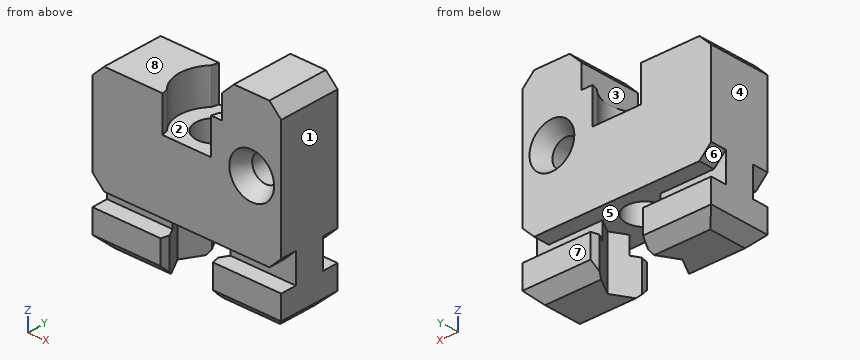
from build123d import *
from OCP.BRepFilletAPI import BRepFilletAPI_MakeChamfer

# Parameters (mm, degrees)
SKETCH1_R           = 1.15
BOSS_EXTRUDE1_DEPTH = 2.6
BOSS_EXTRUDE2_DEPTH = 16
SKETCH3_R           = 1.6
CUT_EXTRUDE1_DEPTH  = 24.13028318
SKETCH4_R           = 3
CUT_EXTRUDE2_DEPTH  = 3
CUT_EXTRUDE3_REACH  = 25.13
CHAMFER1_SIZE       = 0.549227511
CHAMFER1_SIZE_2     = 0.549038106
CHAMFER1_SIZE_3     = 0.75
CHAMFER2_SIZE       = 1
CHAMFER3_SIZE       = 0.75
CHAMFER3_SIZE2      = 1.299038106


with BuildPart() as part:
    # Sketch1 → Boss-Extrude1 (new, symmetric)
    with BuildSketch(Plane(origin=(0, 0, 0), x_dir=(1, 0, 0), z_dir=(0, 1, 0))):
        Polygon((0, 0), (16, 0), (16, -12), (11, -12), (11, -9), (0, -9), align=None)
        with Locations(Location((13.5, -6, 0), (0, 0, 270))):
            Circle(SKETCH1_R, mode=Mode.SUBTRACT)
    extrude(amount=BOSS_EXTRUDE1_DEPTH, both=True)

    # Sketch2 → Boss-Extrude2 (add)
    with BuildSketch(Plane.ZY):
        Polygon((-1.5, -1.25), (-1.5, -2.6), (-4.5, -2.6), (-4.5, 2.6), (-1.5, 2.6), (-1.5, 1.25), (0, 1.25), (0, -1.25), align=None)
    extrude(amount=-BOSS_EXTRUDE2_DEPTH)

    # Sketch3 → Cut-Extrude1 (cut, through all)
    with BuildSketch(Plane(origin=(0, 0, -4.5), x_dir=(-1, 0, 0), z_dir=(0, 0, -1))):
        with Locations((-8, 0)):
            Circle(SKETCH3_R)
    extrude(amount=-CUT_EXTRUDE1_DEPTH, mode=Mode.SUBTRACT)

    # Sketch4 → Cut-Extrude2 (cut)
    with BuildSketch(Plane.XY.offset(9)):
        with Locations((8, 0)):
            Circle(SKETCH4_R)
    extrude(amount=-CUT_EXTRUDE2_DEPTH, mode=Mode.SUBTRACT)

    # Cut-Extrude3: up to this face of the body (flat: up to its plane)
    cut_extrude3_end = Plane(part.part.faces().sort_by_distance((8, 1.937058452, 0))[0])
    # Sketch5 → Cut-Extrude3 (cut, up to the picked face)
    with BuildSketch(Plane(origin=(0, 0, -4.5), x_dir=(-1, 0, 0), z_dir=(0, 0, -1)), mode=Mode.PRIVATE) as cut_extrude3_sk1:
        Polygon((-4.824573519, 0), (-6.41228676, 2.75), (-9.58771324, 2.75), (-11.175426481, 0), (-9.58771324, -2.75), (-6.41228676, -2.75), align=None)
    cut_extrude3_tool1 = split(extrude(cut_extrude3_sk1.sketch, amount=-CUT_EXTRUDE3_REACH, mode=Mode.PRIVATE), bisect_by=cut_extrude3_end, keep=Keep.BOTH, mode=Mode.PRIVATE)
    add(cut_extrude3_tool1.solids().sort_by(Axis((8, 0, -4.5), (0, 0, 1)))[0], mode=Mode.SUBTRACT)

    # Chamfer1
    # the kernel refuses this chamfer: 0.75, 0.549227511, 0.549038106 mm, written as the material it takes off along each edge
    with BuildSketch(Plane(origin=(9.496662955, 2.6, 6), x_dir=(0.7827857508590854, -0.6222913049786071, 0), z_dir=(0, 0, 1)), Plane(origin=(6.503337045, -2.6, 6), x_dir=(-0.7827857508590857, 0.6222913049786067, 0), z_dir=(0, 0, 1))) as chamfer1_piece_1:
        with BuildLine():
            Line((0.892781916, 0), (CHAMFER1_SIZE * 0.782785751548, CHAMFER1_SIZE * 0.622291305526))
            Line((CHAMFER1_SIZE * 0.782785751548, CHAMFER1_SIZE * 0.622291305526), (0, 0))
            ThreePointArc((0, 0), (0.458630217, 0.033371738), (0.892781916, 0))
        make_face()
    extrude(amount=5.292721472, mode=Mode.SUBTRACT)
    with BuildSketch(Plane(origin=(9.496662955, -2.6, 6), x_dir=(0.7827857508590856, 0.6222913049786071, 0), z_dir=(0, 0, 1)), Plane(origin=(6.503337045, 2.6, 6), x_dir=(-0.7827857508590856, -0.622291304978607, 0), z_dir=(0, 0, 1))) as chamfer1_piece_2:
        with BuildLine():
            Line((0.892781916, 0), (CHAMFER1_SIZE * 0.782785751548, -CHAMFER1_SIZE * 0.622291305526))
            Line((CHAMFER1_SIZE * 0.782785751548, -CHAMFER1_SIZE * 0.622291305526), (0, 0))
            ThreePointArc((0, 0), (0.458630217, -0.033371738), (0.892781916, 0))
        make_face()
    extrude(amount=5.292721472, mode=Mode.SUBTRACT)
    with BuildSketch(Plane(origin=(6.325684219, -2.6, -6.428762241), x_dir=(-1, 0, 0), z_dir=(0, 0, 1)), Plane(origin=(9.674315781, -2.6, -1.5), x_dir=(1, 0, 0), z_dir=(0, 0, -1)), Plane(origin=(9.674315781, 2.6, -6.428762241), x_dir=(1, 0, 0), z_dir=(0, 0, 1)), Plane(origin=(6.325684219, 2.6, -1.5), x_dir=(-1, 0, 0), z_dir=(0, 0, -1))) as chamfer1_piece_3:
        Polygon((CHAMFER1_SIZE_2, 0), (CHAMFER1_SIZE_3 * 0.5, -CHAMFER1_SIZE_3 * 0.866025403784), (0, 0), align=None)
    extrude(amount=4.928762241, mode=Mode.SUBTRACT)

    # Chamfer2
    chamfer2_edges = [part.edges().sort_by_distance(p)[0] for p in [
        (16, 0, 12),
        (11, 0, 12),
        (0, 0, 9),
        (16, -1.925, 0),
        (16, 1.925, 0),
        (0, -1.925, 0),
        (0, 1.925, 0),
        (2.888323057, -2.6, -4.5),
        (0, 0, -4.5),
        (16, 0, -4.5),
        (2.888323057, 2.6, -4.5),
        (13.111676943, -2.6, -4.5),
        (13.111676943, 2.6, -4.5),
    ]]
    chamfer(chamfer2_edges, length=CHAMFER2_SIZE)

    # Chamfer3: one chamfer whose edges measure the first distance from different faces: ONE call of the kernel's chamfer builder (chamfer() names one face for all edges)
    chamfer3_edges_1 = [part.edges().sort_by_distance(p)[0] for p in [
        (13.5, -2.6, 4.85),
    ]]
    chamfer3_side_1 = [part.faces().sort_by_distance(p)[0] for p in [
        (8.413951701, -2.6, 4.798840105),
    ]]
    chamfer3_edges_2 = [part.edges().sort_by_distance(p)[0] for p in [
        (13.5, 2.6, 4.85),
    ]]
    chamfer3_side_2 = [part.faces().sort_by_distance(p)[0] for p in [
        (8.413951701, 2.6, 4.798840105),
    ]]
    chamfer3 = BRepFilletAPI_MakeChamfer(part.part.solid().wrapped)
    for e in chamfer3_edges_1:
        chamfer3.Add(CHAMFER3_SIZE, CHAMFER3_SIZE2, e.wrapped, chamfer3_side_1[0].wrapped)  # the first distance lies on this face
    for e in chamfer3_edges_2:
        chamfer3.Add(CHAMFER3_SIZE, CHAMFER3_SIZE2, e.wrapped, chamfer3_side_2[0].wrapped)  # the first distance lies on this face
    add(Compound.cast(chamfer3.Shape()), mode=Mode.REPLACE)


solid = part.part
Geometry check sheet. Reference: the model listing, model coordinates, mm. Face numbers are marked on the shaded views. A direction names the side the tool comes from. Give positions to 0.01 mm unless a question says otherwise; leave off trailing zeros. Write each loop counter-clockwise with the first axis right and the second up, starting at its lowest first coordinate (ties: lowest second). Pieces come first, ordered by that corner, then holes. Notation, with made-up numbers: (-7, 10) - (26, 10) arc R7 ccw to (26, 15) - close; hole circle Ø2 at (-17.75, 42). An arc over 180 degrees is marked (long way). Put each result on its own line as item: value.
1. Go/stop test with flat-tipped pins: pin 1 (0.8 mm diameter, centred on x = 1.5, z = -0.5, fed in from -Y); pin 2 (2.5 mm diameter, centred on x = 6.5, y = 0, fed in from +Z); pin 3 (0.6 mm diameter, centred on y = 0, z = 10, fed in from -X). Record where each tip stops, or that it passes through.
Ans:
pin 1: stops at y = -1.25
pin 2: stops at z = 6
pin 3: stops at x = 11
2. Sectioned sample at A-A, the plane z = -0.75. Enter the section's corners in (x, y).
Ans:
outline: (0, -1.25) - (5.55, -1.25) - (4.82, 0) - (5.55, 1.25) - (0, 1.25) - close; (10.45, -1.25) - (16, -1.25) - (16, 1.25) - (10.45, 1.25) - (11.18, 0) - close
3. Thickness scan on line 1 (X direction, y = 0, z = 1.65); line 2 (Z direction, x = 10.75, y = -1.35); line 3 (Y direction, x = 8, z = 1.35). Record the ranges inside material, lowest first.
Ans:
line 1: x = 0 to 6.4, 9.6 to 16
line 2: z = -4.5 to -1.5, 0 to 9
line 3: y = -2.6 to -1.6, 1.6 to 2.6
4. Sectioned sample at C-C, the plane x = 4.5. Enter the section's corners in (y, z), plus the area to 4 significant figures.
Ans:
outline: (-2.6, -3.5) - (-1.6, -4.5) - (1.6, -4.5) - (2.6, -3.5) - (2.6, -1.5) - (1.25, -1.5) - (1.25, 0) - (2.6, 0) - (2.6, 9) - (-2.6, 9) - (-2.6, 0) - (-1.25, 0) - (-1.25, -1.5) - (-2.6, -1.5) - close
area: 65.15 mm²
5. Sectioned sample at D-D, the plane x = 8. Enter the section's corners in (y, z).
Ans:
outline: (-2.6, 0) - (-1.6, 0) - (-1.6, 6) - (-2.6, 6) - close; (1.6, 0) - (2.6, 0) - (2.6, 6) - (1.6, 6) - close
6. Sectioned sample at B-B, the plane x = 13.5. Enter the section's corners in (y, z).
Ans:
outline: (-2.6, -3.5) - (-1.6, -4.5) - (1.6, -4.5) - (2.6, -3.5) - (2.6, -1.5) - (1.25, -1.5) - (1.25, 0) - (2.6, 0) - (2.6, 4.1) - (1.3, 4.85) - (-1.3, 4.85) - (-2.6, 4.1) - (-2.6, 0) - (-1.25, 0) - (-1.25, -1.5) - (-2.6, -1.5) - close; (-2.6, 7.9) - (-1.3, 7.15) - (1.3, 7.15) - (2.6, 7.9) - (2.6, 12) - (-2.6, 12) - close
7. Set-up check for the marked faces 1, 2, 3, 4 and 5: record each of +Z, -Z, +X, -X, +Y, -Y from which the full face is reachable in a straight line by a thin tool's end or side.
Ans:
face 1: +Z, -Z, +X, +Y, -Y
face 2: +Z
face 3: +Z, -X, +Y, -Y
face 4: +Z, -Z, -X, +Y, -Y
face 5: none
8. Draft check along Z on the marked faces 6, 7 and 8. Enter one of: +Z half, -Z half, draft (parallel to the pull), parting line (faces both ways), or undercut.
Ans:
face 6: undercut
face 7: draft
face 8: +Z half
